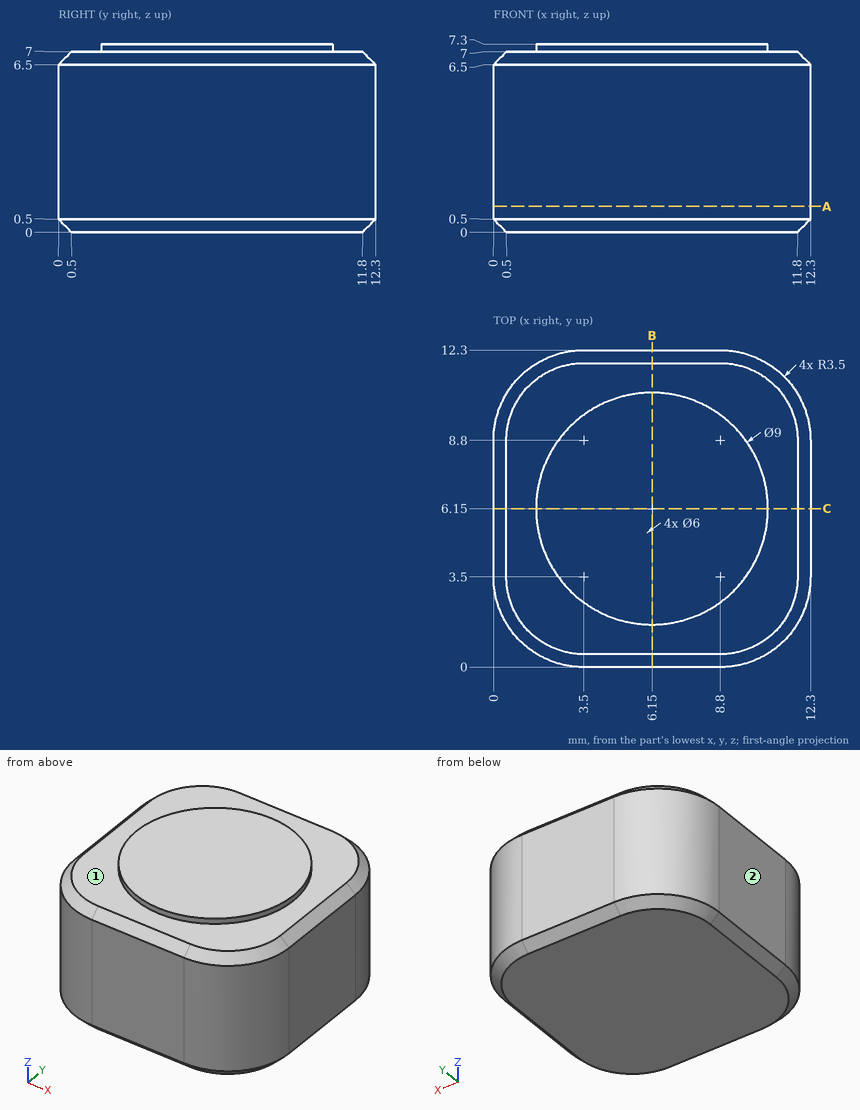
Geometry check sheet. Reference: drawing and pictorial views, mm from the part's lowest x, y, z. A direction names the side the tool comes from. Give positions to 0.01 mm unless a question says otherwise; leave off trailing zeros. Order: outer loops, then holes, each group sorted by start corner. A loop starts at its lowest first (then second) coordinate and runs counter-clockwise, first axis right, second up. Notation, with made-up numbers: M -26,27.25 L -18,27.25 A9 ccw -18,35.25 Z; hole C 27.25,56.5 d9. An arc over 180 degrees is marked long. Use one line per item in the form item = value. Start each with the question number.
Q1. Section check B-B (x = 6.15). Enter the section's corners in (y, z), then the cut area to 3 significant figures.
Q2. Access from +Z, -Z, +X, -X, +Y, -Y to the whole of each face (thin tool, end or side, straight path). Record for the marked faces 1 and 2.
Q3. Scan lines: line 1 along Z through (x, y) = (10, 1.75); line 2 along X through (y, z) = (11.25, 5.75); line 3 along Y through (x, z) = (0.5, 4.75). Record each from-to range of solid material in increasing order. Write a range as [from, to].
Q4. Section check A-A (z = 1). Enter the section's corners in (x, y).
Evaluation:
q1.outline = M 0,0.5 L 0.5,0 L 11.8,0 L 12.3,0.5 L 12.3,6.5 L 11.8,7 L 10.65,7 L 10.65,7.3 L 1.65,7.3 L 1.65,7 L 0.5,7 L 0,6.5 Z
q1.area = 88.3 mm2
q2.face_1 = +Z
q2.face_2 = +Z, -Z, -X, +Y, -Y
q3.line_1 = [0, 7]
q3.line_2 = [1, 11.3]
q3.line_3 = [1.7, 10.6]
q4.outline = M 0,3.5 A3.5 ccw 3.5,0 L 8.8,0 A3.5 ccw 12.3,3.5 L 12.3,8.8 A3.5 ccw 8.8,12.3 L 3.5,12.3 A3.5 ccw 0,8.8 Z
